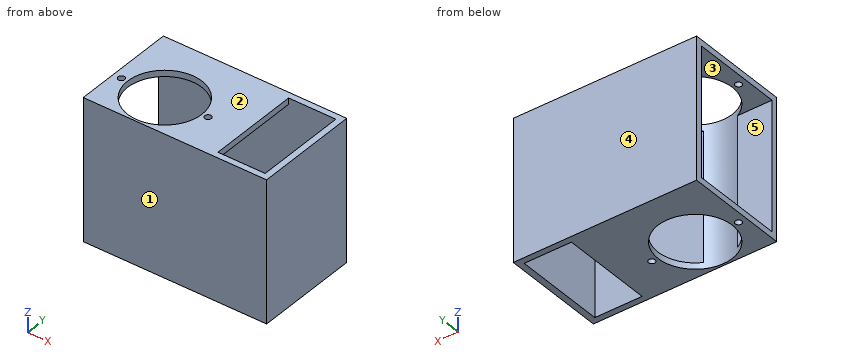
```python
from build123d import *

# Parameters (mm, degrees)
SKETCH1_W           = 88.9
SKETCH1_H           = 50.8
BOSS_EXTRUDE1_DEPTH = 68.58
SHELL10_T           = 3
SKETCH2_R           = 18
SKETCH2_R_2         = 1.6
SKETCH2_W           = 22.9
SKETCH2_H           = 44.8
CUT_EXTRUDE1_DEPTH  = 69
SKETCH4_W           = 62.58
SKETCH4_H           = 44.8
CUT_EXTRUDE2_DEPTH  = 10


with BuildPart() as part:
    # Sketch1 → Boss-Extrude1 (new body)
    with BuildSketch(Plane.XY):
        with Locations((44.45, 25.4)):
            Rectangle(SKETCH1_W, SKETCH1_H)
    extrude(amount=BOSS_EXTRUDE1_DEPTH)

    # Shell10 (no face opened: a closed hollow body)
    add(offset(amount=-SHELL10_T, mode=Mode.PRIVATE), mode=Mode.SUBTRACT)

    # Sketch2 → Cut-Extrude1 (cut)
    with BuildSketch(Plane.XY.offset(68.58)):
        with Locations((25, 19)):
            Circle(SKETCH2_R)
        with Locations((4, 19)):
            Circle(SKETCH2_R_2)
        with Locations(Location((46, 19, 0), (0, 0, 180))):
            Circle(SKETCH2_R_2)
        with Locations((74.45, 25.4)):
            Rectangle(SKETCH2_W, SKETCH2_H)
    extrude(amount=-CUT_EXTRUDE1_DEPTH, mode=Mode.SUBTRACT)

    # Sketch4 → Cut-Extrude2 (cut)
    with BuildSketch(Plane.ZY):
        with Locations((34.29, 25.4)):
            Rectangle(SKETCH4_W, SKETCH4_H)
    extrude(amount=-CUT_EXTRUDE2_DEPTH, mode=Mode.SUBTRACT)


solid = part.part
```
CAD build for the part. Positions are in the model's coordinates, mm. Face numbers are marked on the shaded views. A direction names the side the tool comes from. Round coordinates to 2 decimals unless told otherwise and drop trailing zeros. Order: outer loops, then holes, each group sorted by start corner. A loop starts at its lowest first (then second) coordinate and runs counter-clockwise, first axis right, second up.
Item 1: Saw through at A-A on x = 73.5. Write the cut outline in (y, z).
Item 2: Saw through at B-B on x = 59. Write the cut outline in (y, z).
Item 3: Mould opens along Z. For the marked faces 1, 2 and 3 say: pulls with the +Z half, pulls with the -Z half, needs draft (parallel to the pull), parting line crosses it, or undercut.
Item 4: Tool access for the marked faces 4 and 5: list every direction of +Z, -Z, +X, -X, +Y, -Y with a clear straight run to the whole face (end or side of a thin tool).
Item 5: Probe line 1 along X through (y, z) = (19, 0.95); line 2 along Y through (x, z) = (4, 2.3); line 3 along Y through (x, z) = (25, 47). List the from-to ranges inside material, lowest first.
Item 6: Pin check, flat tips, straight feed: pin 1 (1 mm diameter, centred on y = 42, z = 13, fed in from -X); pin 2 (8 mm diameter, centred on x = 28, z = 57.5, fed in from -Y); pin 3 (2.5 mm diameter, centred on x = 4, y = 19, fed in from -Z). Stop position of each tip, or through.
Item 7: Saw through at C-C on y = 46. Write the cut outline in (x, z), then the cut area to 3 significant figures.
Item 8: Saw through at D-D on z = 46. Write the cut outline in (x, y).
Reported:
1. outline: (0, 0) - (3, 0) - (3, 68.58) - (0, 68.58) - close; (47.8, 0) - (50.8, 0) - (50.8, 68.58) - (47.8, 68.58) - close
2. outline: (0, 0) - (50.8, 0) - (50.8, 68.58) - (0, 68.58) - close; hole (3, 3) - (47.8, 3) - (47.8, 65.58) - (3, 65.58) - close
3. face 1: needs draft
3. face 2: pulls with the +Z half
3. face 3: undercut
4. face 4: +Z, -Z, +X, -X, +Y
4. face 5: -X
5. line 1: x = 0 to 2.4, 5.6 to 7, 43 to 44.4, 47.6 to 63, 85.9 to 88.9
5. line 2: y = 0 to 17.4, 20.6 to 50.8
5. line 3: y = 0 to 1, 47.8 to 50.8
6. pin 1: stops at x = 85.9
6. pin 2: stops at y = 0
6. pin 3: passes through
7. outline: (0, 0) - (63, 0) - (63, 3) - (0, 3) - close; (0, 65.58) - (63, 65.58) - (63, 68.58) - (0, 68.58) - close; (85.9, 0) - (88.9, 0) - (88.9, 68.58) - (85.9, 68.58) - close
7. area: 584 mm2
8. outline: (0, 0) - (88.9, 0) - (88.9, 50.8) - (0, 50.8) - (0, 47.8) - (85.9, 47.8) - (85.9, 3) - (33.25, 3) arc R18 cw to (16.75, 3) - (0, 3) - close
